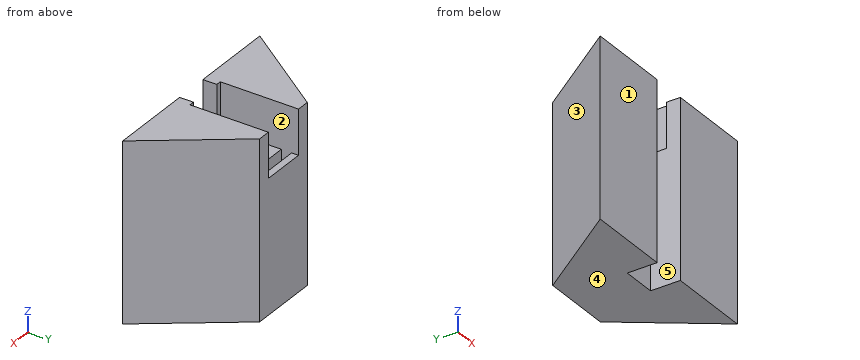
```python
from build123d import *

# Parameters (mm, degrees)
F1_DEPTH = 51.5
F2_W     = 13
F2_H     = 13
F3_DEPTH = 22.75
F4_W     = 13
F4_H     = 3
F5_DEPTH = 5
F6_W     = 10
F6_H     = 8.67
F7_DEPTH = 51.5


with BuildPart() as f1:
    # F0 (on Top) → F1 (new body)
    with BuildSketch(Plane.XY):
        Polygon((-10.25, 13.39471), (-29.5, -13.3945), (29.5, -13.3945), (10.25, 13.39471), align=None)
    extrude(amount=-F1_DEPTH)

    # F2 (on face) → F3 (cut)
    with BuildSketch(Plane(origin=(0, 13.39471, 0), x_dir=(-1, 0, 0), z_dir=(0, 1, 0))):
        with Locations((0, -6.5)):
            Rectangle(F2_W, F2_H)
    extrude(amount=-F3_DEPTH, mode=Mode.SUBTRACT)

    # F4 (on face) → F5 (cut)
    with BuildSketch(Plane.XY.offset(-13)):
        with Locations((0, 9.89471)):
            Rectangle(F4_W, F4_H)
    extrude(amount=-F5_DEPTH, mode=Mode.SUBTRACT)

    # F6 (on face) → F7 (cut)
    with BuildSketch(Plane.XY):
        with Locations((0, -9.0595)):
            Rectangle(F6_W, F6_H)
    extrude(amount=-F7_DEPTH, mode=Mode.SUBTRACT)


solid = f1.part
```
Model file for the job. Use its own axes, mm. Face numbers are marked on the shaded views. A direction names the side the tool comes from. Coordinates: 2 decimals unless noted, no trailing zeros. Order: outer loops, then holes, each group sorted by start corner. A loop starts at its lowest first (then second) coordinate and runs counter-clockwise, first axis right, second up. Notation, with made-up numbers: (-18, 78.25) -> (41, 78.25) arc R15 cw to (41, 99.25) -> close; hole circle Ø10 at (5, 87.25). An arc over 180 degrees is marked (long way). Answer as a JSON object with one key per item and string values. Group by question number.
1) Which spindle directions (+Z, -Z, +X, -X, +Y, -Y) get a long thin tool onto all of the face, cutting with end or side? Do the marked faces 4 and 5. Say none if no direction does.
2) Cut at C-C, the plane x = 2.5. Write the cut outline in (y, z).
3) Cut at A-A, the plane z = -11.5. Write the cut outline in (x, y), then the cut area to 3 significant figures.
4) Cut at D-D, the plane z = -41. Write the cut outline in (x, y), then the cut area to 3 significant figures.
5) Cut at B-B, the plane y = -10.75. Write the cut outline in (x, z).
6) Drill centre lines: L1, parallel to Z at x = -5, y = -4.5; L2, parallel to Y at x = 2, z = -46; L3, parallel to X at y = -7.5, z = -44.5. Where is each one in solid material? Low to high.
7) Flat gauge pins, fed straight in: pin 1 (9 mm diameter, centred on y = 1.5, z = -9, fed in from +X); pin 2 (7 mm diameter, centred on y = -9, z = -29.5, fed in from -X); pin 3 (4.5 mm diameter, centred on y = -10.5, z = -19.5, fed in from +X); pin 4 (1.5 mm diameter, centred on x = 12.5, y = 0.5, fed in from +Z). Where does each tip first touch, or does it go through?
8) Pull direction X, two halves, no side cores. Call the marked faces 1, 2 and 3: +X half, -X half, draft (parallel to the pull), parting line (faces both ways), or undercut.
Check values:
{
 "1": {"face 4": "-Z, +X, -X, +Y, -Y", "face 5": "+Z, -Z, -Y"},
 "2": {"outline": "(-4.72, -51.5) -> (13.39, -51.5) -> (13.39, -13) -> (11.39, -13) -> (11.39, -18) -> (8.39, -18) -> (8.39, -13) -> (-4.72, -13) -> close"},
 "3": {"outline": "(-29.5, -13.39) -> (-5, -13.39) -> (-5, -9.36) -> (-6.5, -9.36) -> (-6.5, 13.39) -> (-10.25, 13.39) -> close; (5, -13.39) -> (29.5, -13.39) -> (10.25, 13.39) -> (6.5, 13.39) -> (6.5, -9.36) -> (5, -9.36) -> close", "area": "729 mm²"},
 "4": {"outline": "(-29.5, -13.39) -> (-5, -13.39) -> (-5, -4.72) -> (5, -4.72) -> (5, -13.39) -> (29.5, -13.39) -> (10.25, 13.39) -> (-10.25, 13.39) -> close", "area": "978 mm²"},
 "5": {"outline": "(-27.6, -51.5) -> (-5, -51.5) -> (-5, 0) -> (-27.6, 0) -> close; (5, -51.5) -> (27.6, -51.5) -> (27.6, 0) -> (5, 0) -> close"},
 "6": {"L1": "z = -51.5 to -13", "L2": "y = -4.72 to 13.39", "L3": "x = -25.26 to -5, 5 to 25.26"},
 "7": {"pin 1": "stops at x = 22.03", "pin 2": "stops at x = -28.86", "pin 3": "stops at x = 29.04", "pin 4": "stops at z = 0"},
 "8": {"face 1": "draft", "face 2": "undercut", "face 3": "-X half"}
}
